For this review, take the finished solid that the model builds, in its own axes (mm). A direction names the side the tool comes from. Round coordinates to 2 decimals unless told otherwise and drop trailing zeros. Order: outer loops, then holes, each group sorted by start corner. A loop starts at its lowest first (then second) coordinate and runs counter-clockwise, first axis right, second up. Notation, with made-up numbers: (52, -40) - (110, -40) arc R8 cw to (110, -32) - close; hole circle Ø7 at (40.5, 49.5). An arc over 180 degrees is marked (long way). One line per item, written item: value.
```python
from build123d import *

# Parameters (mm, degrees)
F0_W     = 6
F0_H     = 5
F1_DEPTH = 15
F2_W     = 10.5033244736
F2_H     = 51.3265209893
F3_DEPTH = 3
F4_W     = 10.5033244736
F4_H     = 52.3007216553
F5_DEPTH = 3
F6_W     = 3
F6_H     = 49.6023270358
F7_DEPTH = 25.4


with BuildPart() as f1:
    # F0 (on Front) → F1 (new body)
    with BuildSketch(Plane.XZ):
        Polygon((-22.9482755264, 10.603449295), (-22.9482755264, -4.396550705), (-16.9482755264, -4.396550705), (-16.9482755264, 5.603449295), (-16.9482755264, 10.603449295), align=None)
        Polygon((4.0517244736, -29.082685709), (4.0517244736, -27.1280445158), (2.7775244736, -27.1280445158), align=None)
        Polygon((4.0517244736, -31.0373269022), (4.0517244736, -29.082685709), (2.7775244736, -29.082685709), align=None)
        Polygon((4.0517244736, -32.9919680953), (4.0517244736, -31.0373269022), (2.7775244736, -31.0373269022), align=None)
        Polygon((4.0517244736, -34.9466092885), (4.0517244736, -32.9919680953), (2.7775244736, -32.9919680953), align=None)
        Polygon((4.0517244736, -36.9012504816), (4.0517244736, -34.9466092885), (2.7775244736, -34.9466092885), align=None)
        Polygon((4.0517244736, -38.8558916748), (4.0517244736, -36.9012504816), (2.7775244736, -36.9012504816), align=None)
        Polygon((4.0517244736, -40.8105328679), (4.0517244736, -38.8558916748), (2.7775244736, -38.8558916748), align=None)
        Polygon((4.0517244736, -42.7651740611), (4.0517244736, -40.8105328679), (2.7775244736, -40.8105328679), align=None)
        Polygon((2.7775244736, -42.7651740611), (4.0517244736, -44.7198152542), (4.0517244736, -42.7651740611), align=None)
        Polygon((2.7775244736, -44.7198152542), (4.0517244736, -46.6744564474), (4.0517244736, -44.7198152542), align=None)
        Polygon((2.7775244736, -46.6744564474), (4.0517244736, -48.6290976405), (4.0517244736, -46.6744564474), align=None)
        Polygon((2.7775244736, -48.6290976405), (4.0517244736, -50.5837388337), (4.0517244736, -48.6290976405), align=None)
        Polygon((2.7775244736, -50.5837388337), (4.0517244736, -52.5383800268), (4.0517244736, -50.5837388337), align=None)
        Polygon((2.7775244736, -52.5383800268), (4.0517244736, -54.49302122), (4.0517244736, -52.5383800268), align=None)
        Polygon((2.7775244736, -54.49302122), (4.0517244736, -56.4476624131), (4.0517244736, -54.49302122), align=None)
        Polygon((2.7775244736, -56.4476624131), (4.0517244736, -58.4023036063), (4.0517244736, -56.4476624131), align=None)
        Polygon((2.7775244736, -58.4023036063), (4.0517244736, -60.3569447994), (4.0517244736, -58.4023036063), align=None)
        with Locations((-13.9482755264, 8.103449295)):
            Rectangle(F0_W, F0_H)
        Polygon((10.5033244736, -13.5344793896), (-4.9482755264, 10.603449295), (-4.9482755264, -13.5344793896), align=None)
        Polygon((4.0517244736, -25.1734033227), (4.0517244736, -23.2300292701), (2.7775244736, -23.2300292701), (4.0443796011, -25.1734033227), align=None)
        Polygon((4.0517244736, -27.1280445158), (4.0517244736, -25.1846704632), (4.0443796011, -25.1734033227), (2.7775244736, -25.1734033227), align=None)
        Polygon((-10.9482755264, 10.603449295), (-10.9482755264, 5.603449295), (-10.9482755264, -19.396550705), (-4.9482755264, -19.396550705), (-4.9482755264, -13.5344793896), (-4.9482755264, 10.603449295), align=None)
        Polygon((-4.9482755264, -13.5344793896), (-4.9482755264, -19.396550705), (4.0517244736, -19.396550705), (10.5033244736, -19.396550705), (10.5033244736, -13.5344793896), align=None)
        Polygon((4.0517244736, -25.1846704632), (4.0517244736, -25.1734033227), (4.0443796011, -25.1734033227), align=None)
        Polygon((10.5033244736, -19.396550705), (4.0517244736, -19.396550705), (4.0517244736, -23.2300292701), (4.0517244736, -25.1734033227), (4.0517244736, -25.1846704632), (4.0517244736, -27.1280445158), (4.0517244736, -29.082685709), (4.0517244736, -31.0373269022), (4.0517244736, -32.9919680953), (4.0517244736, -34.9466092885), (4.0517244736, -36.9012504816), (4.0517244736, -38.8558916748), (4.0517244736, -40.8105328679), (4.0517244736, -42.7651740611), (4.0517244736, -44.7198152542), (4.0517244736, -46.6744564474), (4.0517244736, -48.6290976405), (4.0517244736, -50.5837388337), (4.0517244736, -52.5383800268), (4.0517244736, -54.49302122), (4.0517244736, -56.4476624131), (4.0517244736, -58.4023036063), (4.0517244736, -60.3569447994), (9.7408400844, -68.9988777408), (10.5033244736, -68.9988777408), align=None)
    extrude(amount=F1_DEPTH)

    # F2 (on face) → F3 (cut)
    with BuildSketch(Plane(origin=(0, 0, 0), x_dir=(-1, 0, 0), z_dir=(0, 1, 0))):
        with Locations((-5.2516622368, -45.0598111997)):
            Rectangle(F2_W, F2_H)
    extrude(amount=-F3_DEPTH, mode=Mode.SUBTRACT)

    # F4 (on face) → F5 (cut)
    with BuildSketch(Plane.XZ.offset(15)):
        with Locations((5.2516622368, -45.5469115327)):
            Rectangle(F4_W, F4_H)
    extrude(amount=-F5_DEPTH, mode=Mode.SUBTRACT)

    # F6 (on face) → F7 (cut)
    with BuildSketch(Plane.YZ.offset(10.5033244736)):
        with Locations((-7.5, -44.1977142229)):
            Rectangle(F6_W, F6_H)
    extrude(amount=-F7_DEPTH, mode=Mode.SUBTRACT)


solid = f1.part
```
Item 1: The part is to be moulded in two halves that separate along Z. For faces 1 (the flat face through (3.406, -10.479, -49.593)), 2 (the flat face through (2.886, -7.395, -1.634)), 3 (the flat face through (-6, -15, -4)), say which applies: +Z half, -Z half, draft (parallel to the pull), parting line (faces both ways), or undercut.
Returned:
face 1: undercut
face 2: +Z half
face 3: draft
Item 2: For P1, Ø1.4, axis at x = 3.5, y = -11, coming from the +Z side; P2, Ø2, axis at x = -1, y = -3.5, coming from the -Z side; P3, Ø6, axis at x = 2.5, y = -12, coming from the -Z side, all flat-tipped, find the tip position at first contact; note any pin that passes through.
Returned:
P1: z = -1.5
P2: z = -19.4
P3: z = -62.56
Item 3: Wall thickness on line 1 (Y direction, x = 5.5, z = -30); line 2 (Z direction, x = -9, y = -9); line 3 (Z direction, x = -19, y = -14): over which ranges is each line inside the solid? List them lowest first.
Returned:
line 1: -12 to -9, -6 to -3
line 2: -19.4 to 10.6
line 3: -4.4 to 10.6
Item 4: Take a section at C-C (z = -3). Write out the cut boundary in (x, y), plus the area to 3 significant figures.
Returned:
outline: (-22.95, -15) - (-16.95, -15) - (-16.95, 0) - (-22.95, 0) - close; (-10.95, -15) - (3.76, -15) - (3.76, 0) - (-10.95, 0) - close
area: 311 mm^2
Item 5: Take a section at B-B (y = -13). Write out the cut boundary in (x, z).
Returned:
outline: (-22.95, -4.4) - (-16.95, -4.4) - (-16.95, 5.6) - (-10.95, 5.6) - (-10.95, -19.4) - (10.5, -19.4) - (10.5, -13.53) - (-4.95, 10.6) - (-22.95, 10.6) - close
Item 6: Take a section at A-A (z = -34). Write out the cut boundary in (x, y).
Returned:
outline: (3.43, -12) - (10.5, -12) - (10.5, -9) - (3.43, -9) - close; (3.43, -6) - (10.5, -6) - (10.5, -3) - (3.43, -3) - close
Item 7: Machinability: for faces 4 (the flat face through (8, -6, -45)), 5 (the flat face through (7, -12, -44)), which of the approach directions +Z, -Z, +X, -X, +Y, -Y give a long, thin tool a straight path to every point of the face, cutting with its end or side? Answer none if there is none.
Returned:
face 4: -Z, +X, -X
face 5: -Z, +X, -X, -Y
Item 8: Take a section at D-D (x = -3). Write out the cut boundary in (y, z), plus the area to 3 significant figures.
Returned:
outline: (-15, -19.4) - (0, -19.4) - (0, 7.56) - (-15, 7.56) - close
area: 404 mm^2
